Build history of the part. All positions in model axes, mm. Face numbers are marked on the shaded views. A direction names the side the tool comes from. Round coordinates to 2 decimals unless told otherwise and drop trailing zeros. Write each loop counter-clockwise with the first axis right and the second up, starting at its lowest first coordinate (ties: lowest second). Pieces come first, ordered by that corner, then holes. Notation, with made-up numbers: M 5.25,51.5 L 25.25,51.5 A17 ccw 25.25,64.5 Z; hole C 0,71.5 d11. An arc over 180 degrees is marked long. Use a Markdown table: item, result.
from build123d import *

# Parameters (mm, degrees)
SKETCH1_W                 = 146.259710098
SKETCH1_H                 = 81.954365634
BOSS_EXTRUDE1_DEPTH       = 1
BOSS_EXTRUDE3_DEPTH       = 30
SKETCH3_R                 = 8.932317163
BOSS_EXTRUDE4_DEPTH       = 30
CHAMFER2_SIZE             = 7
CHAMFER2_SIZE2            = 15.722257417
SKETCH5_R                 = 0.765790516
BOSS_EXTRUDE5_DEPTH       = 10
BOSS_EXTRUDE10_DEPTH      = 82.756209
BOSS_EXTRUDE11_DEPTH      = 5
BOSS_EXTRUDE11_DEPTH_BACK = 85
CUT_EXTRUDE1_REACH        = 58.766
SKETCH9_W                 = 8.019759774
SKETCH9_H                 = 10.43964337


with BuildPart() as part:
    # Sketch1 → Boss-Extrude1 (new body)
    with BuildSketch(Plane(origin=(0, 0, 0), x_dir=(1, 0, 0), z_dir=(0, 1, 0))):
        with Locations((4.257398588, 4.671362068)):
            Rectangle(SKETCH1_W, SKETCH1_H)
    extrude(amount=BOSS_EXTRUDE1_DEPTH)

    # Sketch2 → Boss-Extrude3 (add)
    with BuildSketch(Plane(origin=(0, 1, 0), x_dir=(1, 0, 0), z_dir=(0, 1, 0))):
        with BuildLine():
            Line((49.289390862, 31.61533336), (49.289390862, -11.117740331))
            Line((49.289390862, -11.117740331), (-33.466817923, -11.117740331))
            Line((-33.466817923, -11.117740331), (-33.466817923, 17.014992699))
            ThreePointArc((-33.466817923, 17.014992699), (-44.839654232, 27.770758355), (-29.665757449, 31.61533336))
            Line((-29.665757449, 31.61533336), (49.289390862, 31.61533336))
        make_face()
        with BuildLine():
            Line((-31.384885653, 21.995593928), (-31.384885653, -8.380062495))
            Line((-31.384885653, -8.380062495), (47.074717384, -8.380062495))
            Line((47.074717384, -8.380062495), (47.074717384, 28.596341433))
            Line((47.074717384, 28.596341433), (-31.086300879, 28.596341433))
            ThreePointArc((-31.086300879, 28.596341433), (-42.153064375, 25.789819421), (-31.384885653, 21.995593928))
        make_face(mode=Mode.SUBTRACT)
    extrude(amount=BOSS_EXTRUDE3_DEPTH)

    # Sketch3 → Boss-Extrude4 (add)
    with BuildSketch(Plane(origin=(0, 31, 0), x_dir=(1, 0, 0), z_dir=(0, 1, 0))):
        with Locations((-36.195473967, 25.520327854)):
            Circle(SKETCH3_R)
    extrude(amount=BOSS_EXTRUDE4_DEPTH)

    # Chamfer2
    chamfer2_edges = [part.edges().sort_by_distance(p)[0] for p in [
        (-45.12779113, 61, -25.520327854),
    ]]
    chamfer2_side = [part.faces().sort_by_distance(p)[0] for p in [
        (-36.195473967, 61, -25.520327854),
    ]]
    chamfer(chamfer2_edges, length=CHAMFER2_SIZE, length2=CHAMFER2_SIZE2, reference=chamfer2_side[0])

    # Sketch5 → Boss-Extrude5 (add)
    with BuildSketch(Plane(origin=(0, 61, 0), x_dir=(1, 0, 0), z_dir=(0, 1, 0))):
        with Locations((-36.195473967, 25.520327854)):
            Circle(SKETCH5_R)
    extrude(amount=BOSS_EXTRUDE5_DEPTH)

    # Sketch7 → Boss-Extrude10 (add)
    with BuildSketch(Plane(origin=(49.289390862, 0, 0), x_dir=(0, 0, -1), z_dir=(1, 0, 0))):
        Polygon((-11.117740331, 31), (12.411619963, 41.835751537), (31.61533336, 31), align=None)
    extrude(amount=-BOSS_EXTRUDE10_DEPTH)

    # Sketch8 → Boss-Extrude11 (add, two sides)
    with BuildSketch(Plane(origin=(49.289390862, 0, 0), x_dir=(0, 0, -1), z_dir=(1, 0, 0))) as boss_extrude11_sk:
        Polygon((-11.117740331, 31), (12.411619963, 41.835751537), (31.61533336, 31), (33.773667087, 29.849066987), (33.773667087, 31.638529108), (12.411619963, 43.882217303), (-14.672774477, 30.545550786), (-14.672774477, 29.330586748), align=None)
    extrude(amount=BOSS_EXTRUDE11_DEPTH)
    extrude(boss_extrude11_sk.sketch, amount=-BOSS_EXTRUDE11_DEPTH_BACK)

    # Sketch9 → Cut-Extrude1 (cut, up to next)
    with BuildSketch(Plane.XY.offset(11.117740331), mode=Mode.PRIVATE) as cut_extrude1_sk1:
        with Locations((-20.260430368, 6.219821685)):
            Rectangle(SKETCH9_W, SKETCH9_H)
    cut_extrude1_tool1 = extrude(cut_extrude1_sk1.sketch, amount=-CUT_EXTRUDE1_REACH, mode=Mode.PRIVATE) & part.part
    add(cut_extrude1_tool1.solids().sort_by_distance((-20.26043, 6.219822, 11.11774))[0], mode=Mode.SUBTRACT)


solid = part.part
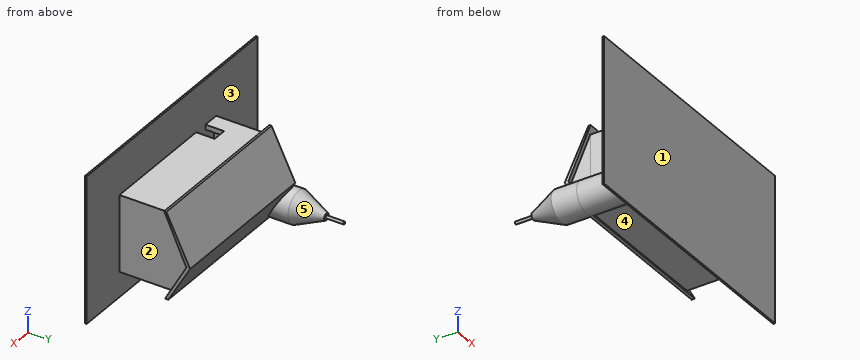
Q1. Cut at B-B on y = 25. Give the cut face in (x, z) (3 decimals).
Response values:
| item | result |
|---|---|
| outline | M -33.467,-17.015 A8.932 ccw long -29.666,-31.615 L 49.289,-31.615 L 49.289,11.118 L -33.467,11.118 Z; hole M -31.385,-21.996 A5.964 ccw long -31.086,-28.596 L 47.075,-28.596 L 47.075,8.38 L -31.385,8.38 Z |
Q2. Drill centre lines: L1, parallel to Z at x = 33.5, y = 26; L2, parallel to X at y = 9, z = -5; L3, parallel to Y at x = -63, z = 32. Where is each one in solid material? Low to high.
Response values:
| item | result |
|---|---|
| L1 | z = -31.62 to -28.6, 8.38 to 11.12 |
| L2 | x = -33.47 to -31.38, 47.07 to 49.29 |
| L3 | y = 0 to 1 |
Q3. Two-plate mould, pull along X, no slides. Class the marked faces 3, 4 and 5: +X half, -X half, draft (parallel to the pull), parting line (faces both ways), or undercut.
Response values:
| item | result |
|---|---|
| face 3 | undercut |
| face 4 | draft |
| face 5 | parting line |
Q4. Cut at D-D on x = -22. Give the cut face in (y, z), and give its area (3 significant figures).
Response values:
| item | result |
|---|---|
| outline | M 0,-45.65 L 1,-45.65 L 1,-31.62 L 31,-31.62 L 29.85,-33.77 L 31.64,-33.77 L 43.88,-12.41 L 30.55,14.67 L 29.33,14.67 L 31,11.12 L 11.44,11.12 L 11.44,8.38 L 31,8.38 L 31,-28.6 L 1,-28.6 L 1,36.31 L 0,36.31 Z |
| area | 543 mm2 |
Q5. Cut at A-A on x = -5. Give the cut face in (y, z), and give its area (3 significant figures).
Response values:
| item | result |
|---|---|
| outline | M 0,-45.65 L 1,-45.65 L 1,-31.62 L 31,-31.62 L 29.85,-33.77 L 31.64,-33.77 L 43.88,-12.41 L 30.55,14.67 L 29.33,14.67 L 31,11.12 L 1,11.12 L 1,36.31 L 0,36.31 Z; hole M 1,-28.6 L 31,-28.6 L 31,8.38 L 1,8.38 Z |
| area | 572 mm2 |
Q6. Cut at C-C on z = -14.5. Give the cut face in (x, y).
Response values:
| item | result |
|---|---|
| outline | M -68.87,0 L 77.39,0 L 77.39,1 L 49.29,1 L 49.29,40.66 L 54.29,40.66 L 54.29,42.69 L -35.71,42.69 L -35.71,40.66 L -33.47,40.66 L -33.47,1 L -68.87,1 Z; hole M -31.38,1 L 47.07,1 L 47.07,31 L -31.38,31 Z |
Q7. Which spindle directions (+Z, -Z, +X, -X, +Y, -Y) get a long thin tool onto all of the face, cutting with end or side? Do the marked faces 1 and 2. Say none if no direction does.
Response values:
| item | result |
|---|---|
| face 1 | +Z, -Z, +X, -X, -Y |
| face 2 | +X |
Q8. Drop flat-ended pins along their axis: P1, Ø1.5, axis at x = 43.5, z = -4.5, coming from the +Y side; P2, Ø24, axis at y = 15.5, z = -5.5, coming from the -X side; P3, Ø3.5, axis at y = 38, z = -7, coming from the -X side. Give the stop position or say it passes through.
Response values:
| item | result |
|---|---|
| P1 | stops at y = 40.36 |
| P2 | stops at x = -40.13 |
| P3 | stops at x = -35.71 |
